Verification items for the finished model (mm, model axes). A direction names the side the tool comes from. Coordinates: 2 decimals unless noted, no trailing zeros. Loops run counter-clockwise (first coordinate to the right, second up) from the corner with the lowest first, then second, coordinate; pieces in that order, holes last. Notation, with made-up numbers: (6.25, -7) -> (45.25, -7) arc R31 cw to (45.25, 22) -> close; hole circle Ø6 at (6.5, -28). An arc over 180 degrees is marked (long way). Answer as a JSON object with one key per item and string values. Group by question number.
Q1. Cross-section at C-C on x = 151. Record the boundary of the cut face in (y, z).
Q2. Cross-section at A-A on y = -22. Record the boundary of the cut face in (x, z).
Q3. Scan lines: L1, parallel to Z at x = 149.5, y = -21.5; L2, parallel to Z at x = 126, y = -17.75; L3, parallel to X at y = -22, z = 91. Record each from-to range of solid material in increasing order.
Q4. Release check for a two-part mould opening along X. For faces 4 (the cylindrical face through (61.711, -17.675, 59.304)), 5 (the flat face through (160, -26, 38)), 6 (the flat face through (111, -25, 44)) record: released by +X, released by -X, zero draft, split by the parting line, or undercut.
Q5. Cross-section at B-B on z = 81.5. Record the boundary of the cut face in (x, y), and give its area (3 significant figures).
Q6. Cross-section at D-D on y = -2.25. Record the boundary of the cut face in (x, z).
Q7. Gauge pin test, flat ends, axial feed: pin 1 Ø8 at (x, y) = (113.5, -15.5) entering from -Z; pin 2 Ø9.5 at (x, z) = (107.5, 43.5) entering from +Y; pin 3 Ø11 at (y, z) = (-26.5, 44) entering from +X. Record the tip position at first contact, or that the pin passes through.
Q8. Set-up check for faces 1 (the flat face through (111, -23, 38)), 2 (the flat face through (109, -20, 34)), 3 (the cylindrical face through (61.804, -17.675, 100.789)): record each of +Z, -Z, +X, -X, +Y, -Y from which the full face is reachable in a straight line by a thin tool's end or side.
```python
from build123d import *

# Parameters (mm, degrees)
F0_W     = 120
F0_H     = 60
F1_DEPTH = 30
F3_DEPTH = 25
F4_W     = 100
F4_H     = 10
F5_DEPTH = 20
F6_W     = 5
F6_H     = 12
F7_DEPTH = 110.001


with BuildPart() as f1:
    # F0 (on Front) → F1 (new body)
    with BuildSketch(Plane.XZ):
        with Locations((110, 80)):
            Rectangle(F0_W, F0_H)
    extrude(amount=F1_DEPTH)

    # F2 (on face) → F3 (cut)
    with BuildSketch(Plane.XZ.offset(30)):
        with BuildLine():
            Line((66, 57.5), (154, 57.5))
            ThreePointArc((154, 57.5), (158.242641, 59.257359), (160, 63.5))
            Line((160, 63.5), (160, 96.5))
            ThreePointArc((160, 96.5), (158.242641, 100.742641), (154, 102.5))
            Line((154, 102.5), (66, 102.5))
            ThreePointArc((66, 102.5), (61.757359, 100.742641), (60, 96.5))
            Line((60, 96.5), (60, 63.5))
            ThreePointArc((60, 63.5), (61.757359, 59.257359), (66, 57.5))
        make_face()
    extrude(amount=-F3_DEPTH, mode=Mode.SUBTRACT)

    # F4 (on face) → F5 (join)
    with BuildSketch(Plane(origin=(0, 0, 50), x_dir=(1, 0, 0), z_dir=(0, 0, -1))):
        with Locations((110, 25)):
            Rectangle(F4_W, F4_H)
    extrude(amount=F5_DEPTH)

    # F6 (on face) → F7 (cut, through all)
    with BuildSketch(Plane.YZ.offset(160)):
        with Locations((-22.5, 44)):
            Rectangle(F6_W, F6_H)
    extrude(amount=-F7_DEPTH, mode=Mode.SUBTRACT)


solid = f1.part
```
Computed values:
{
 "1": {"outline": "(-30, 30) -> (-20, 30) -> (-20, 38) -> (-25, 38) -> (-25, 50) -> (0, 50) -> (0, 110) -> (-30, 110) -> (-30, 102.5) -> (-5, 102.5) -> (-5, 57.5) -> (-30, 57.5) -> close"},
 "2": {"outline": "(50, 50) -> (170, 50) -> (170, 110) -> (50, 110) -> close; (60, 30) -> (160, 30) -> (160, 38) -> (60, 38) -> close; hole (60, 63.5) arc R6 ccw to (66, 57.5) -> (154, 57.5) arc R6 ccw to (160, 63.5) -> (160, 96.5) arc R6 ccw to (154, 102.5) -> (66, 102.5) arc R6 ccw to (60, 96.5) -> close"},
 "3": {"L1": "z = 30 to 38, 50 to 57.5, 102.5 to 110", "L2": "z = 50 to 57.5, 102.5 to 110", "L3": "x = 50 to 60, 160 to 170"},
 "4": {"face 4": "undercut", "face 5": "released by +X", "face 6": "zero draft"},
 "5": {"outline": "(50, -30) -> (60, -30) -> (60, -5) -> (160, -5) -> (160, -30) -> (170, -30) -> (170, 0) -> (50, 0) -> close", "area": "1,100 mm²"},
 "6": {"outline": "(50, 50) -> (170, 50) -> (170, 110) -> (50, 110) -> close"},
 "7": {"pin 1": "stops at z = 50", "pin 2": "stops at y = -25", "pin 3": "stops at x = 160"},
 "8": {"face 1": "+X, -X, +Y", "face 2": "-Z, +X, -X, +Y", "face 3": "-Y"}
}
